```python
from build123d import *

# Parameters (mm, degrees)
EXTRUDE_1_DEPTH     = 60
SKETCH_2_R          = 13
CUT_EXTRUDE_1_DEPTH = 25
CUT_EXTRUDE_3_REACH = 100.803
SKETCH_3_R          = 8.25
CUT_EXTRUDE_4_REACH = 112.168
SKETCH_4_R          = 10
CUT_EXTRUDE_START   = -12
CUT_EXTRUDE_5_DEPTH = 12


with BuildPart() as part:
    # 草图1 → 凸台-拉伸1 (new body)
    with BuildSketch(Plane.XY):
        with BuildLine():
            Line((-75, 16), (75, 16))
            ThreePointArc((75, 16), (91, 0), (75, -16))
            Line((75, -16), (-75, -16))
            ThreePointArc((-75, -16), (-91, 0), (-75, 16))
        make_face()
    extrude(amount=EXTRUDE_1_DEPTH)

    # 草图2 → 切除-拉伸1 (cut)
    with BuildSketch(Plane.XY.offset(60)):
        with Locations((75, 0)):
            Circle(SKETCH_2_R)
    extrude(amount=-CUT_EXTRUDE_1_DEPTH, mode=Mode.SUBTRACT)

    # 草图3 → 切除-拉伸3 (cut, up to next)
    with BuildSketch(Plane.XY.offset(35), mode=Mode.PRIVATE) as cut_extrude_3_sk1:
        with Locations((75, 0)):
            Circle(SKETCH_3_R)
    cut_extrude_3_tool1 = extrude(cut_extrude_3_sk1.sketch, amount=-CUT_EXTRUDE_3_REACH, mode=Mode.PRIVATE) & part.part
    add(cut_extrude_3_tool1.solids().sort_by_distance((75, 0, 35))[0], mode=Mode.SUBTRACT)

    # 草图4 → 切除-拉伸4 (cut, up to next)
    with BuildSketch(Plane.XY.offset(60), mode=Mode.PRIVATE) as cut_extrude_4_sk1:
        with Locations((-75, 0)):
            Circle(SKETCH_4_R)
    cut_extrude_4_tool1 = extrude(cut_extrude_4_sk1.sketch, amount=-CUT_EXTRUDE_4_REACH, mode=Mode.PRIVATE) & part.part
    add(cut_extrude_4_tool1.solids().sort_by_distance((-75, 0, 60))[0], mode=Mode.SUBTRACT)

    # 草图5 → 切除-拉伸5 (cut)
    with BuildSketch(Plane.XY.offset(60).offset(CUT_EXTRUDE_START)):
        with BuildLine():
            Line((-11, 16), (-11, -16))
            Line((-11, -16), (-75, -16))
            ThreePointArc((-75, -16), (-91, 0), (-75, 16))
            Line((-75, 16), (-11, 16))
        make_face()
    cut_extrude_5 = extrude(amount=CUT_EXTRUDE_5_DEPTH, mode=Mode.SUBTRACT)

    # 镜向1: 切除-拉伸5 across plane
    add(cut_extrude_5.mirror(Plane.XY.offset(30)), mode=Mode.SUBTRACT)


solid = part.part
```
Check sheet for the modelled part. Datum: model origin and axes. Units: mm. A direction names the side the tool comes from. Round coordinates to 2 decimals unless told otherwise and drop trailing zeros. Order: outer loops, then holes, each group sorted by start corner. A loop starts at its lowest first (then second) coordinate and runs counter-clockwise, first axis right, second up.
1) Tool access check on faces 4 (the flat face through (29, 0, 60)), 5 (the flat face through (-50, 0, 12)), 6 (the cylindrical face through (-91, 0, 30)), 7 (the flat face through (-11, 0, 54)), 8 (the cylindrical face through (62.013, 0.572, 47.675)). Record the directions out of +Z, -Z, +X, -X, +Y, -Y that give a thin tool (end or side, any length) a straight path to the whole face; none if there is none.
2) Section check D-D (z = 14). Record the boundary of the cut face in (x, y).
3) Go/stop test with flat-tipped pins: pin 1 Ø9.5 at (x, y) = (-70.5, -6.5) entering from +Z; pin 2 Ø3 at (y, z) = (5, 26) entering from -X; pin 3 Ø2 at (y, z) = (2, 23.5) entering from -X. Record where each tip stops, or that it passes through.
4) Section check B-B (y = 0). Record the boundary of the cut face in (x, z).
5) Section check C-C (x = 72). Record the boundary of the cut face in (y, z).
6) Scan lines: line 1 (X direction, y = -0.5, z = 44); line 2 (Y direction, x = 75, z = 46); line 3 (Y direction, x = -75, z = 28). Record each from-to range of solid material in increasing order.
7) Section check A-A (z = 53). Record the boundary of the cut face in (x, y).
8) Mould release check, pull along X, two halves, no side actions. Record for faces 1 (the cylindrical face through (82.87, 2.48, 17.74)), 2 (the flat face through (-50, 0, 48)), 3 (the flat face through (-11, 0, 6)): +X half, -X half, draft (parallel to the pull), parting line (faces both ways), or undercut.
Result:
1. face 4: +Z, +X, -X, +Y, -Y
1. face 5: -Z, -X, +Y, -Y
1. face 6: +Z, -Z, -X
1. face 7: +Z, -X, +Y, -Y
1. face 8: +Z
2. outline: (-75, -16) - (75, -16) arc R16 ccw to (75, 16) - (-75, 16) arc R16 ccw to start; hole circle Ø20 at (-75, 0); hole circle Ø16.5 at (75, 0)
3. pin 1: stops at z = 48
3. pin 2: stops at x = -90.61
3. pin 3: stops at x = -90.97
4. outline: (-91, 12) - (-85, 12) - (-85, 48) - (-91, 48) - close; (-65, 12) - (-11, 12) - (-11, 0) - (66.75, 0) - (66.75, 35) - (62, 35) - (62, 60) - (-11, 60) - (-11, 48) - (-65, 48) - close; (83.25, 0) - (91, 0) - (91, 60) - (88, 60) - (88, 35) - (83.25, 35) - close
5. outline: (-16, 0) - (-7.69, 0) - (-7.69, 35) - (-12.65, 35) - (-12.65, 60) - (-16, 60) - close; (7.69, 0) - (16, 0) - (16, 60) - (12.65, 60) - (12.65, 35) - (7.69, 35) - close
6. line 1: x = -90.99 to -84.99, -65.01 to 62.01, 87.99 to 90.99
6. line 2: y = -16 to -13, 13 to 16
6. line 3: y = -16 to -10, 10 to 16
7. outline: (-11, -16) - (75, -16) arc R16 ccw to (75, 16) - (-11, 16) - close; hole circle Ø26 at (75, 0)
8. face 1: undercut
8. face 2: draft
8. face 3: -X half
